Can you work these out from the model? Positions are in its coordinate system, mm. A direction names the side the tool comes from. Coordinates: 2 decimals unless noted, no trailing zeros. Loops run counter-clockwise (first coordinate to the right, second up) from the corner with the lowest first, then second, coordinate; pieces in that order, holes last.
```python
from build123d import *

# Parameters (mm, degrees)
SKETCH004_W     = 11.9
SKETCH004_H     = 10
PAD002_DEPTH    = 7
SKETCH005_R     = 1.49
POCKET002_DEPTH = 7.001
SKETCH006_W     = 8.9
SKETCH006_H     = 1.05
POCKET003_DEPTH = 10.001


with BuildPart() as part:
    # Sketch004 → Pad002 (new body)
    with BuildSketch(Plane.XY):
        with Locations((-1.274876, -8.312189)):
            Rectangle(SKETCH004_W, SKETCH004_H)
    extrude(amount=PAD002_DEPTH)

    # Sketch005 → Pocket002 (cut, through all)
    with BuildSketch(Plane.XY.offset(7)):
        with Locations((-2.724876, -8.312189)):
            Circle(SKETCH005_R)
    extrude(amount=-POCKET002_DEPTH, mode=Mode.SUBTRACT)

    # Sketch006 → Pocket003 (cut, through all)
    with BuildSketch(Plane.XZ.offset(13.312189)):
        with Locations((-2.774876, 3.475)):
            Rectangle(SKETCH006_W, SKETCH006_H)
    extrude(amount=-POCKET003_DEPTH, mode=Mode.SUBTRACT)


solid = part.part
```
(1) If I drill on probe 1 along Z at (x, y) = (1.25, -4.25); probe 2 along X at (y, z) = (-9, 1); probe 3 along Y at (x, z) = (-3, 1), over which ranges is the centre line in solid material (lowest first)?
Check values:
probe 1: z = 0 to 2.95, 4 to 7
probe 2: x = -7.22 to -4.05, -1.4 to 4.68
probe 3: y = -13.31 to -9.78, -6.85 to -3.31
(2) I want a section at C-C on x = -3.25. Write out the boundary of the cut face in (y, z), then the cut area to 3 significant figures.
Check values:
outline: (-13.31, 0) - (-9.71, 0) - (-9.71, 2.95) - (-13.31, 2.95) - close; (-13.31, 4) - (-9.71, 4) - (-9.71, 7) - (-13.31, 7) - close; (-6.92, 0) - (-3.31, 0) - (-3.31, 2.95) - (-6.92, 2.95) - close; (-6.92, 4) - (-3.31, 4) - (-3.31, 7) - (-6.92, 7) - close
area: 42.9 mm2
(3) Which directions (+Z, -Z, +X, -X, +Y, -Y) give clear straight access to the entire face, cutting with the end or side of a thin tool? Please do faces 1 (the flat face through (1.675, -8.4, 3.5)), 2 (the cylindrical face through (-3.048, -9.767, 5.521)).
Check values:
face 1: -X, +Y, -Y
face 2: +Z, -Z
(4) If we mould it in two halves opening along Z, with no side actions, what happens to faces 3 (the flat face through (-1, -9, 7)), 4 (the flat face through (-1, -9, 0)), 5 (the flat face through (-1.4, -3.312, 2.7)), 6 (the flat face through (-4, -7, 2.95))? For each: released by +Z, released by -Z, zero draft, split by the parting line, or undercut.
Check values:
face 3: released by +Z
face 4: released by -Z
face 5: zero draft
face 6: undercut
(5) I'm going to push flat-ended pins straight in: pin 1 (1.8 mm diameter, centred on x = -2.72, y = -8.31, fed in from -Z); pin 2 (0.5 mm diameter, centred on y = -7.5, z = 3.5, fed in from -X). Where does each tip first touch, or does it pass through?
Check values:
pin 1: passes through
pin 2: stops at x = 1.68
(6) I want a section at D-D on y = -9.5. Write out the boundary of the cut face in (x, z).
Check values:
outline: (-7.22, 0) - (-3.62, 0) - (-3.62, 2.95) - (-7.22, 2.95) - close; (-7.22, 4) - (-3.62, 4) - (-3.62, 7) - (-7.22, 7) - close; (-1.83, 0) - (4.68, 0) - (4.68, 7) - (-1.83, 7) - (-1.83, 4) - (1.68, 4) - (1.68, 2.95) - (-1.83, 2.95) - close
(7) I want a section at B-B on y = -4.5. Write out the boundary of the cut face in (x, z).
Check values:
outline: (-7.22, 0) - (4.68, 0) - (4.68, 7) - (-7.22, 7) - (-7.22, 4) - (1.68, 4) - (1.68, 2.95) - (-7.22, 2.95) - close
(8) I want a section at A-A on x = 1.5. Write out the boundary of the cut face in (y, z).
Check values:
outline: (-13.31, 0) - (-3.31, 0) - (-3.31, 2.95) - (-13.31, 2.95) - close; (-13.31, 4) - (-3.31, 4) - (-3.31, 7) - (-13.31, 7) - close
